For this review, take the finished solid that the model builds, in its own axes (mm). A direction names the side the tool comes from. Give positions to 0.01 mm unless a question says otherwise; leave off trailing zeros. Loops run counter-clockwise (first coordinate to the right, second up) from the corner with the lowest first, then second, coordinate; pieces in that order, holes last. Notation, with made-up numbers: (16, 80) - (31, 80) arc R28 cw to (31, 106) - close; hole circle Ø1 at (8.25, 65). An arc over 180 degrees is marked (long way). Answer in a Markdown table with one row per item.
```python
from build123d import *

# Parameters (mm, degrees)
F0_R        = 50.25
F1_DEPTH    = 6
F2_DEPTH    = 40
F4_D        = 4.4
F3_W        = 7
F3_H        = 3
F5_DEPTH    = 25
F6_R        = 5
F7_R        = 20
F8_T1_DEPTH = 59.75
F9_SIZE     = 1


# Not quite as in the source:
# - a fillet or chamfer that OpenCascade refuses, or shapes differently, is made with other operations: its cross-section is extruded or revolved along the edge and cut away or added


with BuildPart() as f1:
    # F0 (on Top) → F1 (new body)
    with BuildSketch(Plane.XY):
        with BuildLine():
            ThreePointArc((25, -47.0166194021), (45.6443452138, -27.4254671792), (53.25, 0))
            ThreePointArc((53.25, 0), (-27.4254671792, 45.6443452138), (-25, -47.0166194021))
            ThreePointArc((-25, -47.0166194021), (0, -53.25), (25, -47.0166194021))
        make_face()
        Circle(F0_R, mode=Mode.SUBTRACT)
        with BuildLine():
            ThreePointArc((25, -47.0166194021), (0, -53.25), (-25, -47.0166194021))
            Line((-25, -47.0166194021), (-25, -60))
            Line((-25, -60), (25, -60))
            Line((25, -60), (25, -47.0166194021))
        make_face()
        Polygon((25, -60), (-25, -60), (-25, -65), (0, -65), (25, -65), align=None)
    extrude(amount=F1_DEPTH)

    # F0 (on Top) → F2 (join)
    with BuildSketch(Plane.XY):
        Polygon((25, -60), (-25, -60), (-25, -65), (0, -65), (25, -65), align=None)
    extrude(amount=-F2_DEPTH)

    # F4 (through all)
    with Locations(Plane(origin=(0, -60, 0), x_dir=(-1, 0, 0), z_dir=(0, 1, 0))):
        with Locations((0, -15)):
            Hole(F4_D / 2)

    # F3 (on face) → F5 (cut)
    with BuildSketch(Plane(origin=(0, -60, 0), x_dir=(-1, 0, 0), z_dir=(0, 1, 0))):
        with Locations((-13.5, -31.5)):
            Rectangle(F3_W, F3_H)
        with Locations((13.5, -31.5)):
            Rectangle(F3_W, F3_H)
    extrude(amount=-F5_DEPTH, mode=Mode.SUBTRACT)

    # F6
    f6_edges = [f1.edges().sort_by_distance(p)[0] for p in [
        (-25, -47.016619, 3),
        (25, -47.016619, 3),
        (0, -60, 0),
    ]]
    fillet(f6_edges, radius=F6_R)

    # F7
    f7_edges = [f1.edges().sort_by_distance(p)[0] for p in [
        (25, -62.5, -40),
        (-25, -62.5, -40),
    ]]
    fillet(f7_edges, radius=F7_R)

    # F8: fillet of radius 5 on 2 edges, made by hand

    # F8_s2 → F8_t1 (cut)
    with BuildSketch(Plane.XY.offset(-41.25)):
        with BuildLine():
            ThreePointArc((25, -60), (23.5355339059, -63.5355339059), (20, -65))
            Line((20, -65), (25, -65))
            Line((25, -65), (25, -60))
        make_face()
        with BuildLine():
            ThreePointArc((-20, -65), (-23.5355339059, -63.5355339059), (-25, -60))
            Line((-25, -60), (-25, -65))
            Line((-25, -65), (-20, -65))
        make_face()
    extrude(amount=F8_T1_DEPTH, mode=Mode.SUBTRACT)

    # F9
    f9_edges = [f1.edges().sort_by_distance(p)[0] for p in [
        (-50.25, 0, 0),
    ]]
    chamfer(f9_edges, length=F9_SIZE)


solid = f1.part
```
1. For faces 4 (the face through (25, -55, 3)), 5 (the face through (-13, -62, -33)), 6 (the face through (0, -60, -22)), list the 3-axis set-ups (+Z, -Z, +X, -X, +Y, -Y) from which the entire face can be reached by the end or side of a thin tool; tool diameter is ignored.
Values:
| item | result |
|---|---|
| face 4 | +Z, -Z, +X, -Y |
| face 5 | +Y, -Y |
| face 6 | -Z, +X, -X, +Y |
2. We need section B-B, the plane z = -15. Give the boundary of the cut face in (x, y), and give its area (3 significant figures).
Values:
| item | result |
|---|---|
| outline | (-25, -60) arc R5 ccw to (-20, -65) - (-2.2, -65) - (-2.2, -60) - close; (2.2, -65) - (20, -65) arc R5 ccw to (25, -60) - (2.2, -60) - close |
| area | 217 mm^2 |
3. Clearance check with flat-ended pins moving along their axes: pin 1 (5 mm diameter, centred on y = -53.5, z = -0.5, fed in from +X); pin 2 (5.5 mm diameter, centred on x = 14.5, y = -61.5, fed in from -Z); pin 3 (2.5 mm diameter, centred on y = -62, z = -31, fed in from +X); pin 4 (5.5 mm diameter, centred on x = 0, z = -15, fed in from -Y). State where each tip first meets the part, or that it passes through.
Values:
| item | result |
|---|---|
| pin 1 | stops at x = 25 |
| pin 2 | stops at z = -38.83 |
| pin 3 | stops at x = 22.46 |
| pin 4 | stops at y = -65 |
4. Mouldability with a two-part tool opening along Z and no side actions: class faces 1 (the face through (27.014, 42.371, 3.465)), 2 (the face through (17, -62, -36)), 3 (the face through (-17, -62, -32)) as released by +Z, released by -Z, zero draft, split by the parting line, or undercut.
Values:
| item | result |
|---|---|
| face 1 | zero draft |
| face 2 | released by -Z |
| face 3 | undercut |
5. Wall thickness on line 1 (Z direction, x = 0, y = -62.55); line 2 (Y direction, x = 0, z = 3); line 3 (Y direction, x = 16.5, z = -34.5): over which ranges is each line inside the solid? List them lowest first. Write a range as [from, to].
Values:
| item | result |
|---|---|
| line 1 | z = [-40, -17.2], [-12.8, 6] |
| line 2 | y = [-65, -50.25], [50.25, 53.25] |
| line 3 | y = [-65, -60] |
6. We need section A-A, the plane x = 0. Give the boundary of the cut face in (y, z), and give its area (3 significant figures).
Values:
| item | result |
|---|---|
| outline | (-65, -40) - (-60, -40) - (-60, -17.2) - (-65, -17.2) - close; (-65, -12.8) - (-60, -12.8) - (-60, -5) arc R5 cw to (-55, 0) - (-51.25, 0) - (-50.25, 1) - (-50.25, 6) - (-65, 6) - close; (50.25, 1) - (51.25, 0) - (53.25, 0) - (53.25, 6) - (50.25, 6) - close |
| area | 289 mm^2 |
